The listing builds one solid part. Answer for the finished solid, in the listing's coordinates (mm). Give positions to 0.01 mm unless a question says otherwise; leave off trailing zeros. Order: outer loops, then holes, each group sorted by start corner. A loop starts at its lowest first (then second) coordinate and runs counter-clockwise, first axis right, second up. Notation, with made-up numbers: M 35.25,14.25 L 68.25,14.25 A19 ccw 68.25,21.25 Z; hole C -9,83.5 d3. An arc over 180 degrees is marked long. Answer as a JSON object with one key per item and string values. Group by question number.
```python
from build123d import *

# Parameters (mm, degrees)
F0_R     = 44.95
F1_DEPTH = 3
F2_R     = 1.45
F2_R_2   = 2.5
F3_DEPTH = 3.001
F4_R     = 3
F5_DEPTH = 3.001


with BuildPart() as f1:
    # F0 (on Front) → F1 (new body)
    with BuildSketch(Plane.XZ):
        Circle(F0_R)
    extrude(amount=F1_DEPTH)

    # F2 (on face) → F3 (cut, through all)
    with BuildSketch(Plane.XZ.offset(3)):
        with Locations((-8, 0)):
            Circle(F2_R)
        with Locations((8, 0)):
            Circle(F2_R)
        Circle(F2_R_2)
    extrude(amount=-F3_DEPTH, mode=Mode.SUBTRACT)

    # F4 (on face) → F5 (cut, through all)
    with BuildSketch(Plane.XZ.offset(3)):
        with Locations((-27.5, 27.5)):
            Circle(F4_R)
        with Locations((27.5, 27.5)):
            Circle(F4_R)
        with Locations((-27.5, -27.5)):
            Circle(F4_R)
        with Locations((27.5, -27.5)):
            Circle(F4_R)
    extrude(amount=-F5_DEPTH, mode=Mode.SUBTRACT)


solid = f1.part
```
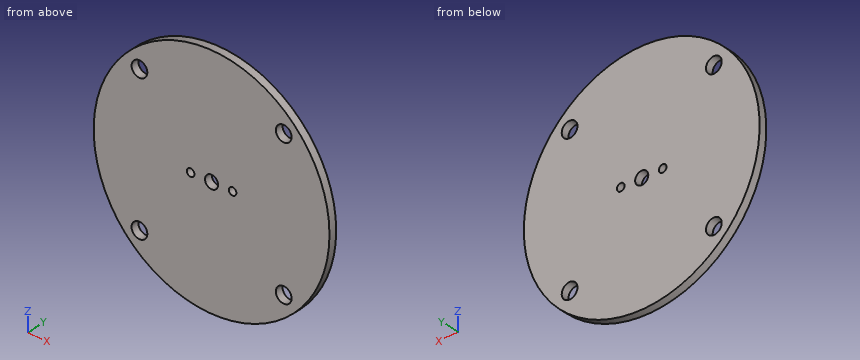
Item 1: Flat-ended cylindrical pins translate along their axes: P1, Ø5, axis at x = -26.5, z = -29, coming from the -Y side; P2, Ø5, axis at x = 27.5, z = 27.5, coming from the +Y side; P3, Ø1, axis at y = -0.5, z = -14, coming from the +X side; P4, Ø1, axis at y = -0.5, z = 13.5, coming from the -X side. Find the tip coordinate at first contact, or state that the pin passes through.
Item 2: Section D-D (z = 27.5) is taken. Determine the outline of the cut face in (x, y).
Item 3: Section C-C (y = -1.9) is taken. Determine the outline of the cut face in (x, z).
Item 4: Section B-B (z = 0) is taken. Determine the outline of the cut face in (x, y), and give its area (3 significant figures).
Item 5: Section A-A (x = 0) is taken. Determine the outline of the cut face in (y, z).
Item 6: Consider probe 1 along Z at (x, y) = (27.5, -2.35); probe 2 along X at (y, z) = (-1.2, 26.5); probe 3 along Z at (x, y) = (-29, -0.65). Determine where each line is inside the solid, lowest interval first. Write a range as from..to.
Values found:
{
 "1": {"P1": "stops at y = -3", "P2": "passes through", "P3": "stops at x = 42.87", "P4": "stops at x = -43.03"},
 "2": {"outline": "M -35.56,-3 L -30.5,-3 L -30.5,0 L -35.56,0 Z; M -24.5,-3 L 24.5,-3 L 24.5,0 L -24.5,0 Z; M 30.5,-3 L 35.56,-3 L 35.56,0 L 30.5,0 Z"},
 "3": {"outline": "C 0,0 d89.9; hole C -27.5,-27.5 d6; hole C -27.5,27.5 d6; hole C -8,0 d2.9; hole C 0,0 d5; hole C 8,0 d2.9; hole C 27.5,-27.5 d6; hole C 27.5,27.5 d6"},
 "4": {"outline": "M -44.95,-3 L -9.45,-3 L -9.45,0 L -44.95,0 Z; M -6.55,-3 L -2.5,-3 L -2.5,0 L -6.55,0 Z; M 2.5,-3 L 6.55,-3 L 6.55,0 L 2.5,0 Z; M 9.45,-3 L 44.95,-3 L 44.95,0 L 9.45,0 Z", "area": "237 mm^2"},
 "5": {"outline": "M -3,-44.95 L 0,-44.95 L 0,-2.5 L -3,-2.5 Z; M -3,2.5 L 0,2.5 L 0,44.95 L -3,44.95 Z"},
 "6": {"probe 1": "z = -35.56..-30.5, -24.5..24.5, 30.5..35.56", "probe 2": "x = -36.31..-30.33, -24.67..24.67, 30.33..36.31", "probe 3": "z = -34.34..-30.1, -24.9..24.9, 30.1..34.34"}
}
